Verification items for the finished model (mm, model axes). Face numbers are marked on the shaded views. Round coordinates to 2 decimals unless told otherwise and drop trailing zeros. Order: outer loops, then holes, each group sorted by start corner. A loop starts at its lowest first (then second) coordinate and runs counter-clockwise, first axis right, second up. Notation, with made-up numbers: M 0.5,50 L 9.5,50 A37 cw 9.5,89 Z; hole C 36.5,-13.75 d11. An arc over 180 degrees is marked long. Use one line per item in the form item = value. Start each with the question number.
Item 1: Cross-section at C-C on z = 1.4. Count the separate pieces of the cut face and the enclosed holes in it, then the cut area to 3 significant figures.
Item 2: Cross-section at A-A on y = -120.5. Enter the section's corners in (x, z).
Item 3: Thickness scan on probe 1 along X at (y, z) = (-203.1, 1.45); probe 2 along X at (y, z) = (-109, 0.3); probe 3 along Y at (x, z) = (34, 1.9). Record the ranges inside material, lowest first. Write a range as [from, to].
Item 4: Cross-section at B-B on x = 56.5. Enter the section's corners in (y, z).
Item 5: Go/stop test with flat-tipped pins: pin 1 Ø10 at (x, y) = (56.5, -102) entering from +Z; pin 2 Ø0.6 at (y, z) = (-79.5, 0.5) entering from +X; pin 3 Ø1 at (y, z) = (-79.5, 1) entering from -X; pin 4 Ø1 at (y, z) = (-99.5, 1.5) entering from -X. Record where each tip stops, or that it passes through.
Item 6: Release check for a two-part mould opening along Z. For the marked faces 1 and 2 record: +Z half, -Z half, draft (parallel to the pull), parting line (faces both ways), or undercut.
from build123d import *

# Parameters (mm, degrees)
SKETCH2_R           = 1.35
SKETCH2_R_2         = 1.5
SKETCH2_R_3         = 1.2
BOSS_EXTRUDE1_DEPTH = 2.1


with BuildPart() as part:
    # Sketch2 → Boss-Extrude1 (new body)
    with BuildSketch(Plane.XY):
        with BuildLine():
            Line((26.360509399, -75.742028439), (106.365509399, -75.742028439))
            Line((106.365509399, -75.742028439), (106.365509399, -82.742028439))
            Line((106.365509399, -82.742028439), (96.904474191, -82.742028439))
            Line((96.904474191, -82.742028439), (81.697018799, -82.742028439))
            ThreePointArc((81.697018799, -82.742028439), (80.282805236, -83.327814877), (79.697018799, -84.742028439))
            Line((79.697018799, -84.742028439), (79.697018799, -123.261425865))
            ThreePointArc((79.697018799, -123.261425865), (80.744039239, -129.647705362), (83.77547538, -135.365328342))
            Line((83.77547538, -135.365328342), (106.022052818, -164.628605146))
            ThreePointArc((106.022052818, -164.628605146), (109.053488959, -170.346228126), (110.100509399, -176.732507623))
            Line((110.100509399, -176.732507623), (110.100509399, -204.994023391))
            ThreePointArc((110.100509399, -204.994023391), (108.636252911, -208.529347679), (105.101102272, -209.994023356))
            Line((105.101102272, -209.994023356), (54.697018799, -210))
            Line((54.697018799, -210), (25.307981201, -210))
            Line((25.307981201, -210), (27.625509399, -210))
            ThreePointArc((27.625509399, -210), (24.089975493, -208.535533906), (22.625509399, -205))
            Line((22.625509399, -205), (22.625509399, -176.738128469))
            ThreePointArc((22.625509399, -176.738128469), (23.672257836, -170.352656272), (26.702934917, -164.635582379))
            Line((26.702934917, -164.635582379), (48.951574482, -135.364417621))
            ThreePointArc((48.951574482, -135.364417621), (51.982251563, -129.647343728), (53.029, -123.261871531))
            Line((53.029, -123.261871531), (53.029, -84.742028439))
            ThreePointArc((53.029, -84.742028439), (52.443213562, -83.327814877), (51.029, -82.742028439))
            Line((51.029, -82.742028439), (37.207455392, -82.742028439))
            Line((37.207455392, -82.742028439), (26.360509399, -82.742028439))
            Line((26.360509399, -82.742028439), (26.360509399, -75.742028439))
        make_face()
        with Locations((46.525509399, -159.877)):
            Circle(SKETCH2_R, mode=Mode.SUBTRACT)
        with Locations((46.525509399, -203.1)):
            Circle(SKETCH2_R, mode=Mode.SUBTRACT)
        with Locations((86.200509399, -203.1)):
            Circle(SKETCH2_R, mode=Mode.SUBTRACT)
        with Locations((86.200509399, -159.877)):
            Circle(SKETCH2_R, mode=Mode.SUBTRACT)
        with Locations((33.106129256, -201)):
            Circle(SKETCH2_R_2, mode=Mode.SUBTRACT)
        with Locations((33.106129256, -177)):
            Circle(SKETCH2_R_2, mode=Mode.SUBTRACT)
        with Locations((99.697018799, -177)):
            Circle(SKETCH2_R_2, mode=Mode.SUBTRACT)
        with Locations((99.697018799, -201)):
            Circle(SKETCH2_R_2, mode=Mode.SUBTRACT)
        with Locations((32.132455392, -79.242028439)):
            Circle(SKETCH2_R_3, mode=Mode.SUBTRACT)
        with Locations((102.282455392, -79.242028439)):
            Circle(SKETCH2_R_3, mode=Mode.SUBTRACT)
        with BuildLine():
            Line((55.129, -82.742028439), (77.597018799, -82.742028439))
            Line((77.597018799, -82.742028439), (77.597018799, -123.261871531))
            add(Edge.make_bspline(
                [(80.187269615, -134.115336952), (77.487014109, -128.558048488), (77.597018799, -123.261871531)],
                knots=[0, 0, 0, 0.393827238, 0.393827238, 0.393827238], degree=2))
            Line((80.187269615, -134.115336952), (94.526314775, -152.977))
            Line((94.526314775, -152.977), (38.202239304, -152.977))
            Line((38.202239304, -152.977), (52.538749184, -134.115336952))
            add(Edge.make_bspline(
                [(52.538749184, -134.115336952), (55.239004689, -128.558048488), (55.129, -123.261871531)],
                knots=[0, 0, 0, 0.393827238, 0.393827238, 0.393827238], degree=2))
            Line((55.129, -123.261871531), (55.129, -82.742028439))
        make_face(mode=Mode.SUBTRACT)
    extrude(amount=BOSS_EXTRUDE1_DEPTH)


solid = part.part
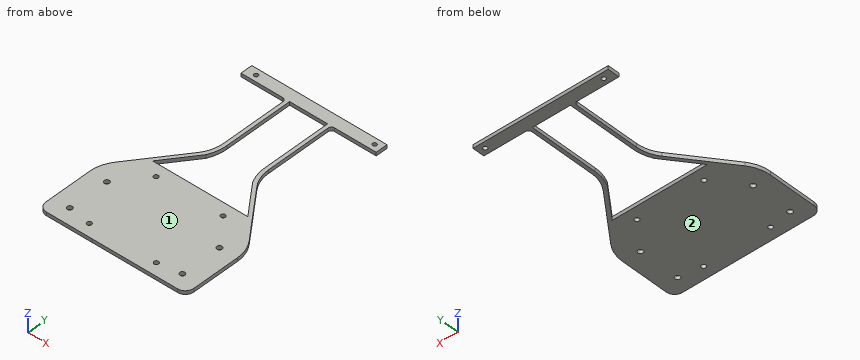
Output values:
q1.separate_pieces = 1
q1.enclosed_holes = 11
q1.area = 5,570 mm2
q2.outline = M 53.03,0 L 55.13,0 L 55.13,2.1 L 53.03,2.1 Z; M 77.6,0 L 79.7,0 L 79.7,2.1 L 77.6,2.1 Z
q3.probe_1 = [22.63, 45.18], [47.88, 84.85], [87.55, 110.1]
q3.probe_2 = [53.03, 55.13], [77.6, 79.7]
q3.probe_3 = [-210, -202.2], [-199.8, -178.2], [-175.8, -155.04], [-82.74, -75.74]
q4.outline = M -210,0 L -152.98,0 L -152.98,2.1 L -210,2.1 Z; M -82.74,0 L -75.74,0 L -75.74,2.1 L -82.74,2.1 Z
q5.pin_1 = 2.1
q5.pin_2 = 106.37
q5.pin_3 = 26.36
q5.pin_4 = 53.03
q6.face_1 = +Z half
q6.face_2 = -Z half
